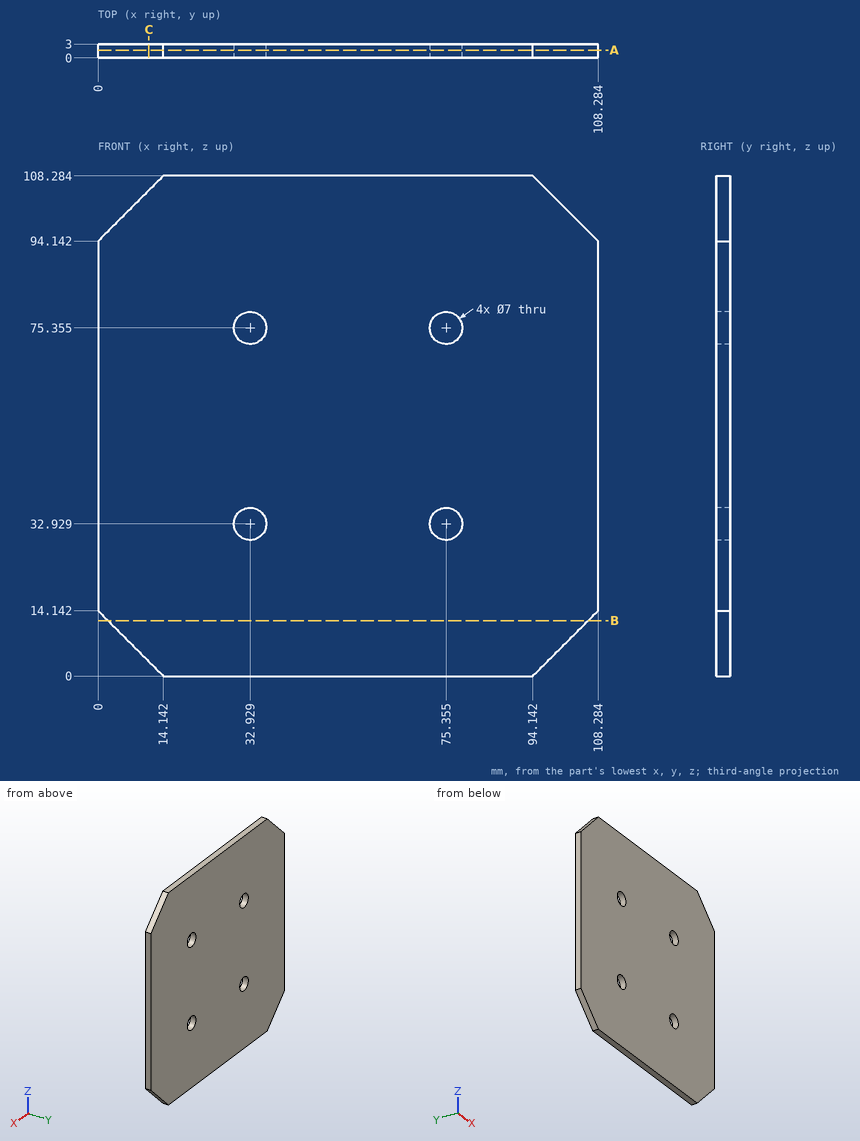
Answer from the drawing. Dimensions are ordinates in mm from the lowest x, y and z of the part. Round coordinates to 2 decimals unless told otherwise and drop trailing zeros. Write each loop counter-clockwise with the first axis right and the second up, starting at its lowest first coordinate (ties: lowest second). Pieces come first, ordered by that corner, then holes. Notation, with made-up numbers: (86, -39) - (105, -39) arc R12 ccw to (105, -28) - close; hole circle Ø2 at (-26.75, -4.5). An arc over 180 degrees is marked (long way). Use a Markdown table: item, result.
(1) The part is cut by section C-C (x = 11). Write down the section's boundary in (y, z), then the cut area to 3 significant figures.
Reported:
| item | result |
|---|---|
| outline | (0, 3.14) - (3, 3.14) - (3, 105.14) - (0, 105.14) - close |
| area | 306 mm2 |
(2) The part is cut by section B-B (z = 12). Write down the section's boundary in (x, y).
Reported:
| item | result |
|---|---|
| outline | (2.14, 0) - (106.14, 0) - (106.14, 3) - (2.14, 3) - close |
(3) The part is cut by section A-A (y = 1.65). Write down the section's boundary in (x, z) (1 decimal).
Reported:
| item | result |
|---|---|
| outline | (0, 14.1) - (14.1, 0) - (94.1, 0) - (108.3, 14.1) - (108.3, 94.1) - (94.1, 108.3) - (14.1, 108.3) - (0, 94.1) - close; hole circle Ø7 at (32.9, 32.9); hole circle Ø7 at (32.9, 75.4); hole circle Ø7 at (75.4, 32.9); hole circle Ø7 at (75.4, 75.4) |
(4) Straight lines are drawn through the part: line 1 along Z through (x, y) = (75, 2.65) (1 decimal); line 2 along X through (y, z) = (2.6, 73) (1 decimal); line 3 along Z through (x, y) = (7, 2.8). For each, find the intervals that lie inside material, in ascending order. Write a range as [from, to].
Reported:
| item | result |
|---|---|
| line 1 | [0, 29.4], [36.4, 71.9], [78.8, 108.3] |
| line 2 | [0, 30.3], [35.5, 72.8], [77.9, 108.3] |
| line 3 | [7.14, 101.14] |
(5) This flat-tipped pin is pushed along its axis until it touches: pin 1 Ø1.5 at (y, z) = (2, 12) entering from -X. Where does it stop, or does it pass through?
Reported:
| item | result |
|---|---|
| pin 1 | x = 1.39 |
